from build123d import *

# Parameters (mm, degrees)
F0_R     = 9.838377
F0_R_2   = 30.041909
F0_R_3   = 9.418189
F1_DEPTH = 25.4


with BuildPart() as f1:
    # F0 (on Front) → F1 (new body)
    with BuildSketch(Plane.XZ):
        with BuildLine():
            Line((73.439807, 60.956387), (-48.24732, 60.956387))
            ThreePointArc((-48.24732, 60.956387), (-66.207833, 53.516899), (-73.64732, 35.556387))
            Line((-73.64732, 35.556387), (-73.64732, -21.692736))
            ThreePointArc((-73.64732, -21.692736), (-66.207833, -39.653248), (-48.24732, -47.092736))
            Line((-48.24732, -47.092736), (73.439807, -47.092736))
            Line((73.439807, -47.092736), (73.439807, 60.956387))
        make_face()
        with Locations((52.279174, -27.384311)):
            Circle(F0_R, mode=Mode.SUBTRACT)
        with Locations((-29.666394, 10.372892)):
            Circle(F0_R_2, mode=Mode.SUBTRACT)
        with Locations((53.316444, 25.102355)):
            Circle(F0_R_3, mode=Mode.SUBTRACT)
    extrude(amount=F1_DEPTH)


solid = f1.part
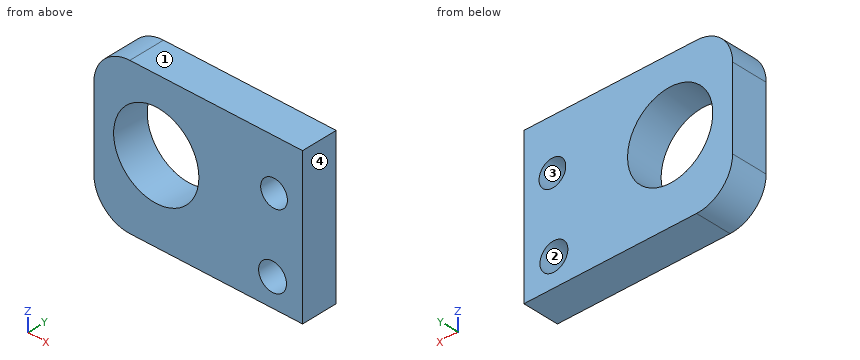
Here's how the part is built. I have some questions about the finished solid (model axes, mm). Face numbers are marked on the shaded views. Round coordinates to 2 decimals unless told otherwise and drop trailing zeros. Loops run counter-clockwise (first coordinate to the right, second up) from the corner with the lowest first, then second, coordinate; pieces in that order, holes last. Notation, with made-up numbers: (-4.5, 60) -> (18.5, 60) arc R31 cw to (18.5, 84) -> close; hole circle Ø2 at (42, 23). An arc over 180 degrees is marked (long way). Write each question's results on one line, items separated by ' | '.
(1) If we section it at C-C, the plane y = -18: List the corners of the cut face in (x, z) for me, then the cut area to 3 significant figures.
Worked answers:
outline: (-73.65, -21.69) arc R25.4 ccw to (-48.25, -47.09) -> (73.44, -47.09) -> (73.44, 60.96) -> (-48.25, 60.96) arc R25.4 ccw to (-73.65, 35.56) -> close; hole circle Ø60.08 at (-29.67, 10.37); hole circle Ø19.68 at (52.28, -27.38); hole circle Ø18.84 at (53.32, 25.1) | area: 12,200 mm2
(2) If I drill on L1, parallel to X at y = -3, z = 9.5; L2, parallel to X at y = -1.25, z = 27.5; L3, parallel to X at y = -12.5, z = 28, over which ranges is the centre line in solid material (lowest first)?
Worked answers:
L1: -73.65 to -59.7, 0.36 to 73.44 | L2: -73.65 to -54.35, -4.98 to 44.21, 62.42 to 73.44 | L3: -73.65 to -53.99, -5.34 to 44.36, 62.28 to 73.44
(3) We'd pull the mould along X, two halves only. Please class the marked faces 1, 2, 3 and 4: released by +X, released by -X, zero draft, split by the parting line, or undercut.
Worked answers:
face 1: zero draft | face 2: undercut | face 3: undercut | face 4: released by +X
(4) If we section it at D-D, the plane z = -2.5: List the corners of the cut face in (x, y) for me, then the cut area to 3 significant figures.
Worked answers:
outline: (-73.65, -25.4) -> (-56.81, -25.4) -> (-56.81, 0) -> (-73.65, 0) -> close; (-2.52, -25.4) -> (73.44, -25.4) -> (73.44, 0) -> (-2.52, 0) -> close | area: 2,360 mm2
(5) If we section it at B-B, the plane z = 31: List the corners of the cut face in (x, y) for me, then the cut area to 3 significant figures.
Worked answers:
outline: (-73.65, -25.4) -> (-51.51, -25.4) -> (-51.51, 0) -> (-73.65, 0) -> close; (-7.83, -25.4) -> (45.97, -25.4) -> (45.97, 0) -> (-7.83, 0) -> close; (60.66, -25.4) -> (73.44, -25.4) -> (73.44, 0) -> (60.66, 0) -> close | area: 2,250 mm2
(6) If we section it at A-A, the plane x = -32: List the corners of the cut face in (y, z) for me, then the cut area to 3 significant figures.
Worked answers:
outline: (-25.4, -47.09) -> (0, -47.09) -> (0, -19.58) -> (-25.4, -19.58) -> close; (-25.4, 40.32) -> (0, 40.32) -> (0, 60.96) -> (-25.4, 60.96) -> close | area: 1,220 mm2
